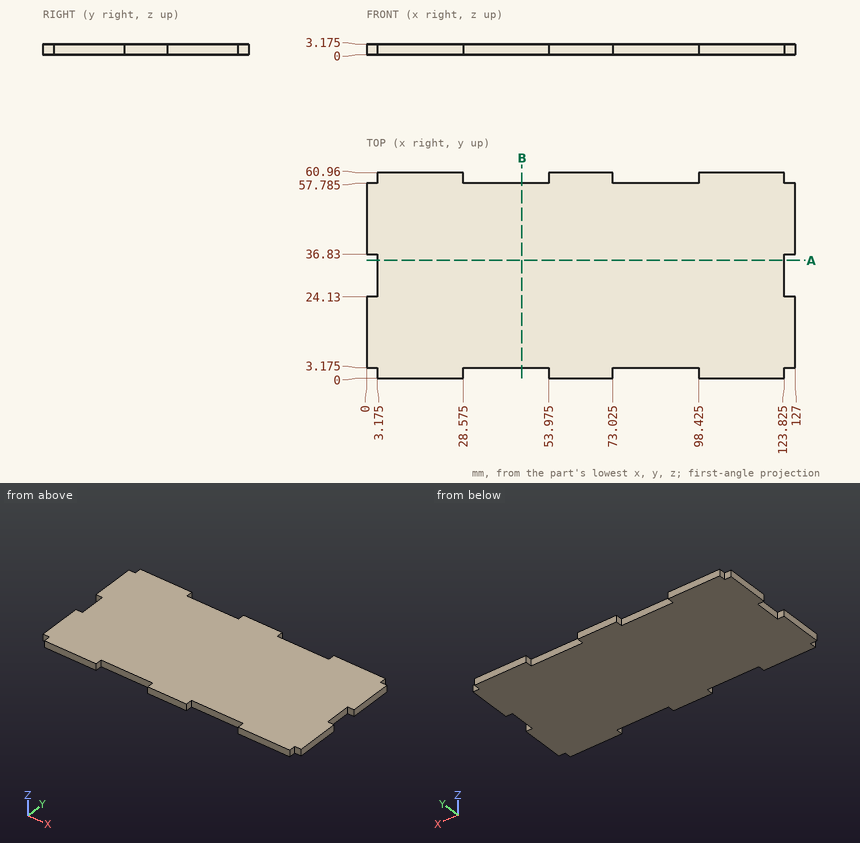
Verification items for this drawing (mm, ordinates from the low corner). Coordinates: 2 decimals unless noted, no trailing zeros. Loops run counter-clockwise (first coordinate to the right, second up) from the corner with the lowest first, then second, coordinate; pieces in that order, holes last.
Item 1: Go/stop test with flat-tipped pins: pin 1 Ø1 at (y, z) = (60, 2) entering from -X (3 decimals); pin 2 Ø1.6 at (y, z) = (59, 2) entering from +X (3 decimals); pin 3 Ø1 at (x, z) = (125, 2) entering from +Y (3 decimals). Record where each tip stops, or that it passes through.
Item 2: Sectioned sample at B-B, the plane x = 46. Record the boundary of the cut face in (y, z) (3 decimals), then the cut area to 3 significant figures.
Item 3: Sectioned sample at A-A, the plane y = 35. Record the boundary of the cut face in (x, z) (3 decimals).
Item 4: Thickness scan on line 1 (Y direction, x = 32, z = 2) (3 decimals); line 2 (X direction, y = 32, z = 1.9) (3 decimals). Record the ranges inside material, lowest first.
Check result:
1. pin 1: stops at x = 3.175
1. pin 2: stops at x = 123.825
1. pin 3: stops at y = 57.785
2. outline: (3.175, 0) - (57.785, 0) - (57.785, 3.175) - (3.175, 3.175) - close
2. area: 173 mm2
3. outline: (3.175, 0) - (123.825, 0) - (123.825, 3.175) - (3.175, 3.175) - close
4. line 1: y = 3.175 to 57.785
4. line 2: x = 3.175 to 123.825
